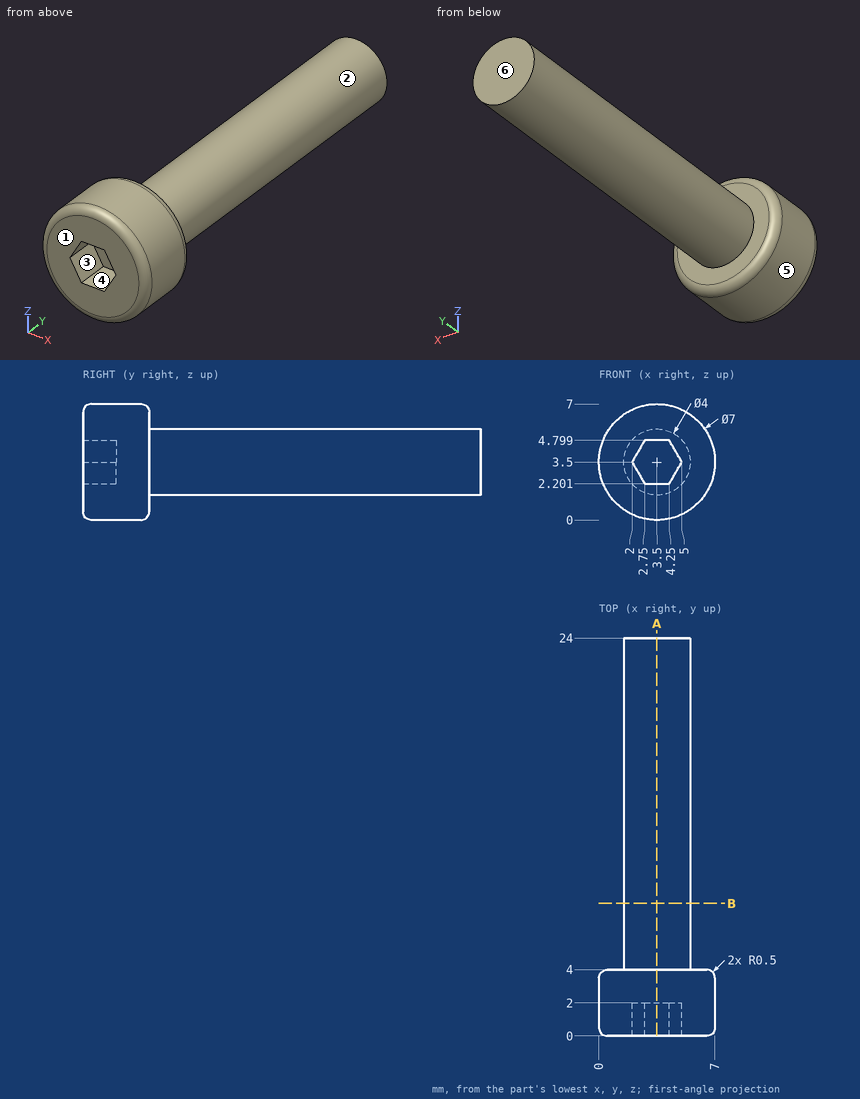
Design review of the part shown in the three views and the two pictorial views. Dimensions are in mm from the part's minimum x, y and z. A direction names the side the tool comes from. Coordinates: 2 decimals unless noted, no trailing zeros. Loops run counter-clockwise (first coordinate to the right, second up) from the corner with the lowest first, then second, coordinate; pieces in that order, holes last. Notation, with made-up numbers: (23.5, 46) - (79.5, 46) arc R20 ccw to (79.5, 69) - close; hole circle Ø10 at (54.25, 62). An arc over 180 degrees is marked (long way). Use a Markdown table: item, result. Add a question column.
Item 1: Insertion check: pin 1 Ø1 at (x, y) = (3, 18) entering from +Z; pin 2 Ø1.3 at (x, z) = (3.5, 3) entering from -Y; pin 3 Ø1.5 at (y, z) = (19.5, 4.5) entering from -X. Each pin has a flat end and moves straight along its axis. Give the tip position at first contact, or say it passes through.
Item 2: Tool access review of the marked faces 1, 2 and 3: name each direction out of +Z, -Z, +X, -X, +Y, -Y from which nothing blocks a thin tool from reaching the whole face with its end or side.
Item 3: We need section A-A (x = 3.5). Give the boundary of the cut face in (y, z), and give its area (3 significant figures).
Item 4: We need section B-B (y = 8). Give the boundary of the cut face in (x, z).
Item 5: Mouldability with a two-part tool opening along X and no side actions: class the marked faces 4, 5 and 6 as pulls with the +X half, pulls with the -X half, needs draft (parallel to the pull), parting line crosses it, or undercut.
Item 6: For line 1 (Y direction, x = 6, z = 2); line 2 (Y direction, x = 2.75, z = 3.25); line 3 (Z direction, x = 3, y = 5.5), list the stretches that pass through material, from the lowest coordinate up.
Results list:
| question | item | result |
|---|---|---|
| 1 | pin 1 | stops at z = 5.5 |
| 1 | pin 2 | stops at y = 2 |
| 1 | pin 3 | stops at x = 1.52 |
| 2 | face 1 | +Z, -Z, +X, -X, -Y |
| 2 | face 2 | +Y |
| 2 | face 3 | -Y |
| 3 | outline | (0, 0.5) arc R0.5 ccw to (0.5, 0) - (3.5, 0) arc R0.5 ccw to (4, 0.5) - (4, 1.5) - (24, 1.5) - (24, 5.5) - (4, 5.5) - (4, 6.5) arc R0.5 ccw to (3.5, 7) - (0.5, 7) arc R0.5 ccw to (0, 6.5) - (0, 4.8) - (2, 4.8) - (2, 2.2) - (0, 2.2) - close |
| 3 | area | 103 mm^2 |
| 4 | outline | circle Ø4 at (3.5, 3.5) |
| 5 | face 4 | undercut |
| 5 | face 5 | parting line crosses it |
| 5 | face 6 | needs draft |
| 6 | line 1 | y = 0 to 4 |
| 6 | line 2 | y = 2 to 24 |
| 6 | line 3 | z = 1.56 to 5.44 |
